Design review of the part built by this model. Coordinates are the model's own, in mm. Coordinates: 2 decimals unless noted, no trailing zeros. Write each loop counter-clockwise with the first axis right and the second up, starting at its lowest first coordinate (ties: lowest second). Pieces come first, ordered by that corner, then holes.
Q1. Add section C-C, the plane z = 1.45. Give the boundary of the cut face in (x, y), plus the area to 3 significant figures.
Q2. To check wall thickness, follow probe 1 along X at (y, z) = (34.72, 2.5); probe 2 along Y at (x, z) = (-60.12, 1.05); probe 3 along X at (y, z) = (42, 2.8). State the ranges of each line that lie inside material, in increasing order.
Q3. Add section D-D, the plane y = 26.72. Give the boundary of the cut face in (x, z), plus the area to 3 significant figures.
Q4. Add section A-A, the plane y = 42.72. Give the boundary of the cut face in (x, z), plus the area to 3 significant figures.
Q5. Add section B-B, the plane x = -60.12. Give the boundary of the cut face in (y, z), plus the area to 3 significant figures.
Q6. Clearance check with flat-ended pins moving along their axes: pin 1 Ø2 at (x, y) = (-35, -36) entering from -Z; pin 2 Ø1.5 at (y, z) = (-29.5, 2.5) entering from +X; pin 3 Ø1.9 at (y, z) = (29.5, 1) entering from +X; pin 4 Ø1 at (y, z) = (-33, 0.5) entering from -X. State where each tip first meets the part, or that it passes through.
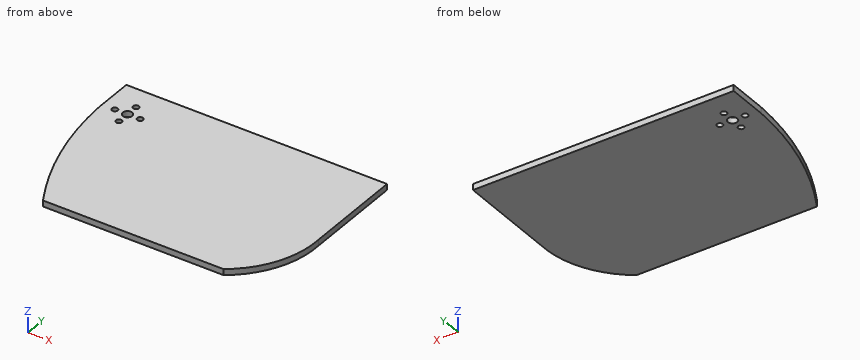
Autodesk Inventor part; units mm, degrees
ref_plane "YZ Plane" through (0, 0, 0) normal (1, 0, 0) x (0, 1, 0)
ref_plane "XZ Plane" through (0, 0, 0) normal (0, 1, 0) x (-1, 0, 0)
ref_plane "XY Plane" through (0, 0, 0) normal (0, 0, 1) x (1, 0, 0)
sketch "Sketch1" plane through (0, 0, 0) normal (0, 0, 1) x (1, 0, 0)
  line L0 (-76.2, 57.15) -> (88.9, 57.15)
  line L1 (88.9, -57.15) -> (-76.2, 57.15) construction
  line L2 (-76.2, -57.15) -> (88.9, 57.15) construction
  line L3 (-76.2, 57.15) -> (-76.2, 31.75)
  arc A0 (-76.2, 31.75) -> (-50.8, -57.15) centre (118.0556, 39.173) ccw
  arc A1 (63.5, -57.15) -> (88.9, -6.35) centre (29.9616, -8.6308) ccw
  line L4 (88.9, 57.15) -> (88.9, -6.35)
  line L5 (63.5, -57.15) -> (-50.8, -57.15)
  point P0 (6.35, 0)
  dimension "d21" = 165.1
  dimension "d22" = 114.3
  dimension "d23" = 25.4
  dimension "d24" = 25.4
  dimension "d25" = 50.8
  dimension "d26" = 25.4
extrude "Extrusion1" add sketch "Sketch1" along normal blind 3.81
sketch "Sketch2" plane through (0, 0, 3.81) normal (0, 0, 1) x (1, 0, 0)
  circle A0 centre (-60.12, 42.72) radius 1.75
  circle A1 centre (-52.12, 34.72) radius 1.75
  circle A2 centre (-68.12, 34.72) radius 1.75
  circle A3 centre (-60.12, 26.72) radius 1.75
  circle A4 centre (-60.12, 34.72) radius 2.85
  point P0 (0, 0)
hole "Hole1" at (-60.12, 42.72, 3.81) at (-68.12, 34.72, 3.81) at (-60.12, 26.72, 3.81) at (-52.12, 34.72, 3.81) direction (0, 0, -1) diameter 3.7 end through all
sketch "Sketch3" plane through (0, 0, 3.81) normal (0, 0, 1) x (1, 0, 0)
  circle A0 centre (-60.12, 34.72) radius 2.85
  point P0 (0, 0)
hole "Hole2" at (-60.12, 34.72, 3.81) direction (0, 0, -1) diameter 6 end through all
properties part number "Bucket - door" material "PET Plastic"
Here are the results:
1. outline: (-76.2, 31.75) arc R194.4 ccw to (-50.8, -57.15) - (63.5, -57.15) arc R58.98 ccw to (88.9, -6.35) - (88.9, 57.15) - (-76.2, 57.15) - close; hole circle Ø3.7 at (-68.12, 34.72); hole circle Ø6 at (-60.12, 34.72); hole circle Ø3.7 at (-60.12, 26.72); hole circle Ø3.7 at (-60.12, 42.72); hole circle Ø3.7 at (-52.12, 34.72)
1. area: 17,600 mm2
2. probe 1: x = -76.2 to -69.97, -66.27 to -63.12, -57.12 to -53.97, -50.27 to 88.9
2. probe 2: y = -38.57 to 24.87, 28.57 to 31.72, 37.72 to 40.87, 44.57 to 57.15
2. probe 3: x = -76.2 to -61.82, -58.42 to 88.9
3. outline: (-75.94, 0) - (-61.97, 0) - (-61.97, 3.81) - (-75.94, 3.81) - close; (-58.27, 0) - (88.9, 0) - (88.9, 3.81) - (-58.27, 3.81) - close
3. area: 614 mm2
4. outline: (-76.2, 0) - (-61.97, 0) - (-61.97, 3.81) - (-76.2, 3.81) - close; (-58.27, 0) - (88.9, 0) - (88.9, 3.81) - (-58.27, 3.81) - close
4. area: 615 mm2
5. outline: (-38.57, 0) - (24.87, 0) - (24.87, 3.81) - (-38.57, 3.81) - close; (28.57, 0) - (31.72, 0) - (31.72, 3.81) - (28.57, 3.81) - close; (37.72, 0) - (40.87, 0) - (40.87, 3.81) - (37.72, 3.81) - close; (44.57, 0) - (57.15, 0) - (57.15, 3.81) - (44.57, 3.81) - close
5. area: 314 mm2
6. pin 1: stops at z = 0
6. pin 2: stops at x = 85.41
6. pin 3: stops at x = 88.9
6. pin 4: stops at x = -62.65
